from build123d import *

# Parameters (mm, degrees)
CUT_EXTRUDE1_DEPTH = 1


with BuildPart() as part:
    # Sketch1 → Revolve1 (revolve)
    with BuildSketch(Plane.XY):
        Polygon((-2, 0), (-2, 1.3125), (-1.8125, 1.5), (0, 1.5), (0, 0.8), (5.7545, 0.8), (6, 0.5545), (6, 0), align=None)
    revolve(axis=Axis((6, 0, 0), (-1, 0, 0)))

    # Sketch2 → Cut-Revolve1 (revolve, cut)
    with BuildSketch(Plane.XY):
        Polygon((-2, 0), (-2, 0.9), (-1.85, 0.75), (-1, 0.75), (-0.6, 0), align=None)
    revolve(axis=Axis((-0.6, 0, 0), (-1, 0, 0)), mode=Mode.SUBTRACT)

    # Sketch3 → Cut-Extrude1 (cut)
    with BuildSketch(Plane(origin=(-2, 0, 0), x_dir=(0, 0, -1), z_dir=(1, 0, 0))):
        Polygon((-0.75, -0.433012702), (0, -0.866025404), (0.75, -0.433012702), (0.75, 0.433012702), (0, 0.866025404), (-0.75, 0.433012702), align=None)
    extrude(amount=CUT_EXTRUDE1_DEPTH, mode=Mode.SUBTRACT)


solid = part.part
Verification items for the finished model (mm, model axes). A direction names the side the tool comes from. Coordinates: 2 decimals unless noted, no trailing zeros. Order: outer loops, then holes, each group sorted by start corner. A loop starts at its lowest first (then second) coordinate and runs counter-clockwise, first axis right, second up. Notation, with made-up numbers: M -33.5,35 L -5.5,35 A13 cw -5.5,39 Z; hole C 2.25,64 d1. An arc over 180 degrees is marked long. One line per item, written item: value. Start each with the question number.
Item 1: Mould release check, pull along Z, two halves, no side actions. Record for faces 1 (the flat face through (0, 0, 1)), 2 (the flat face through (-1.5, 0, 0.75)), 3 (the cylindrical face through (2.92, -0.63, 0.49)): released by +Z, released by -Z, zero draft, split by the parting line, or undercut.
Item 2: Gauge pin test, flat ends, axial feed: pin 1 (1 mm diameter, centred on y = -1, z = 1, fed in from -X); pin 2 (1 mm diameter, centred on x = 3, y = 0.5, fed in from -Z); pin 3 (1.5 mm diameter, centred on x = 2, z = -1, fed in from +Y). Record the tip position at first contact, or that the pin passes through.
Item 3: Access from +Z, -Z, +X, -X, +Y, -Y to the whole of each face (thin tool, end or side, straight path). Record for faces 4 (the cylindrical face through (-0.89, -1.5, -0.07)), 5 (the flat face through (-1.5, 0, -0.75)).
Item 4: Scan lines: probe 1 along X at (y, z) = (-0.55, 1.15); probe 2 along Y at (x, z) = (-0.5, 1.3); probe 3 along Z at (x, y) = (1.75, 0.05). Record each from-to range of solid material in increasing order.
Item 5: Sectioned sample at A-A (x = 2.5). Enter the section's corners in (y, z).
Conclusion:
1. face 1: zero draft
1. face 2: undercut
1. face 3: split by the parting line
2. pin 1: stops at x = -2
2. pin 2: stops at z = -0.8
2. pin 3: stops at y = 0.76
3. face 4: +X, -X
3. face 5: -X
4. probe 1: x = -2 to 0
4. probe 2: y = -0.75 to 0.75
4. probe 3: z = -0.8 to 0.8
5. outline: C 0,0 d1.6
